Verification items for the finished model (mm, model axes). Face numbers are marked on the shaded views. A direction names the side the tool comes from. Coordinates: 2 decimals unless noted, no trailing zeros. Loops run counter-clockwise (first coordinate to the right, second up) from the corner with the lowest first, then second, coordinate; pieces in that order, holes last. Notation, with made-up numbers: (-19.75, 86) -> (31.25, 86) arc R29 cw to (31.25, 107) -> close; hole circle Ø2 at (50.25, -22). An arc over 180 degrees is marked (long way). Answer as a JSON object with one key per item and string values. Group by question number.
Q1. Cross-section at D-D on x = 13.25. Record the boundary of the cut face in (y, z).
Q2. Release check for a two-part mould opening along Y. For the marked faces 4, 5 and 6 record: released by +Y, released by -Y, zero draft, split by the parting line, or undercut.
Q3. Gauge pin test, flat ends, axial feed: pin 1 Ø3 at (x, z) = (12.5, 4.5) entering from -Y; pin 2 Ø1.5 at (x, z) = (4, 2) entering from -Y; pin 3 Ø6 at (x, y) = (0, 0) entering from -Z; pin 4 Ø3 at (x, y) = (-3, 11) entering from +Z. Record the tip position at first contact, or that the pin passes through.
Q4. Cross-section at C-C on y = -9.75. Record the boundary of the cut face in (x, z), and give its area (3 significant figures).
Q5. Cross-section at A-A on x = -1.25. Record the boundary of the cut face in (y, z).
Q6. Cross-section at B-B on z = 1.5. Record the boundary of the cut face in (x, y).
Q7. Set-up check for the marked faces 1, 2 and 3: record each of +Z, -Z, +X, -X, +Y, -Y from which the full face is reachable in a straight line by a thin tool's end or side.
Q8. Scan lines: L1, parallel to X at y = 0, z = 1.7; L2, parallel to Z at x = 8.75, y = -3.75; L3, parallel to X at y = 0.75, z = 2.45. Record each from-to range of solid material in increasing order.
```python
from build123d import *

# Parameters (mm, degrees)
EXTRUDE016_DEPTH = 0.5
ARRAY_COUNT      = 20


with BuildPart() as revolve003:
    # Sketch022 → Revolve003 (revolve)
    with BuildSketch(Plane.XZ):
        Polygon((-3.3, 1), (-15, 1), (-15, 2), (-8, 2), (-8, 6), (-6, 6), (-6, 2), (-3.3, 2), align=None)
    revolve(axis=Axis((0, 0, 0), (0, 0, 1)))


with BuildPart() as barrel003:
    # Sketch023 → Extrude016 (new body, symmetric)
    with BuildSketch(Plane.XZ):
        Polygon((-8, 6), (-15, 2), (-7, 2), (-7, 6), align=None)
    extrude(amount=EXTRUDE016_DEPTH, both=True)

    # Array: barrel003 ×20 about axis
    array_axis = Axis((0, 0, 0), (0, 0, 1))


with BuildPart() as barrel003_1:
    add(barrel003.part)
    for i in range(1, ARRAY_COUNT):
        add(barrel003.part.rotate(array_axis, i * 360 / ARRAY_COUNT))

    # Fusion005: union Revolve003
    add(revolve003.part)


solid = barrel003_1.part
```
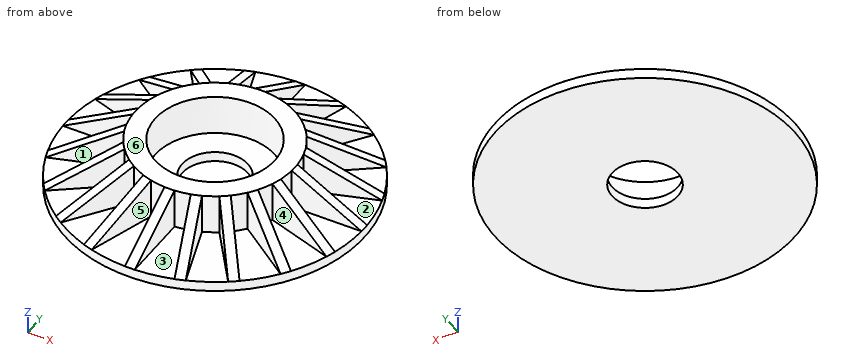
Computed values:
{
 "1": {"outline": "(-7.03, 1) -> (7.03, 1) -> (7.03, 2) -> (4.83, 2) -> (4.83, 2.52) -> (3.78, 2.7) -> (3.78, 2) -> (0.5, 2) -> (0.5, 3) -> (-0.5, 3) -> (-0.5, 2) -> (-3.78, 2) -> (-3.78, 2.7) -> (-4.83, 2.52) -> (-4.83, 2) -> (-7.03, 2) -> close"},
 "2": {"face 4": "undercut", "face 5": "released by -Y", "face 6": "zero draft"},
 "3": {"pin 1": "stops at y = -4.57", "pin 2": "stops at y = -14.64", "pin 3": "passes through", "pin 4": "stops at z = 4.92"},
 "4": {"outline": "(-11.4, 1) -> (11.4, 1) -> (11.4, 2) -> (7.7, 2) -> (7.7, 3.48) -> (6.47, 3.89) -> (6.47, 2) -> (3.69, 2) -> (3.69, 4.62) -> (2.64, 4.81) -> (2.64, 2) -> (0.5, 2) -> (0.5, 5) -> (-0.5, 5) -> (-0.5, 2) -> (-2.64, 2) -> (-2.64, 4.81) -> (-3.69, 4.62) -> (-3.69, 2) -> (-6.47, 2) -> (-6.47, 3.89) -> (-7.7, 3.48) -> (-7.7, 2) -> (-11.4, 2) -> close", "area": "35.7 mm²"},
 "5": {"outline": "(-14.95, 1) -> (-3.05, 1) -> (-3.05, 2) -> (-5.87, 2) -> (-5.87, 6) -> (-7.9, 6) -> (-7.9, 2) -> (-14.95, 2) -> close; (3.05, 1) -> (14.95, 1) -> (14.95, 2) -> (7.9, 2) -> (7.9, 6) -> (5.87, 6) -> (5.87, 2) -> (3.05, 2) -> close"},
 "6": {"outline": "circle Ø30 at (0, 0); hole circle Ø6.6 at (0, 0)"},
 "7": {"face 1": "+Z", "face 2": "+Z, +X", "face 3": "+Z, -Y"},
 "8": {"L1": "x = -15 to -3.3, 3.3 to 15", "L2": "z = 1 to 2", "L3": "x = -7.96 to -5.95, 5.95 to 7.96"}
}
